Check sheet for the modelled part. Datum: model origin and axes. Units: mm. A direction names the side the tool comes from. Round coordinates to 2 decimals unless told otherwise and drop trailing zeros. Order: outer loops, then holes, each group sorted by start corner. A loop starts at its lowest first (then second) coordinate and runs counter-clockwise, first axis right, second up. Notation, with made-up numbers: (36.25, -36) -> (90.25, -36) arc R38 ccw to (90.25, 3) -> close; hole circle Ø5 at (11, 0). An arc over 180 degrees is marked (long way). Answer in a Markdown table with one row per item.
```python
from build123d import *

# Parameters (mm, degrees)
F0_W     = 130
F0_H     = 130
F1_DEPTH = 10
F3_DEPTH = 10
F4_R     = 1.5
F5_DEPTH = 10
F6_R     = 2.5
F7_DEPTH = 10
F8_R     = 3


with BuildPart() as f1:
    # F0 (on Front) → F1 (new body)
    with BuildSketch(Plane.XZ):
        Rectangle(F0_W, F0_H)
    extrude(amount=F1_DEPTH)

    # F2 (on face) → F3 (cut, through all)
    with BuildSketch(Plane.XZ.offset(10)):
        Polygon((8.8, 19.5), (-8.8, 19.5), (-19.5, 8.768557), (-19.5, -8.768557), (-8.8, -19.5), (8.8, -19.5), (19.5, -8.768557), (19.5, 8.768557), align=None)
    extrude(amount=-F3_DEPTH, mode=Mode.SUBTRACT)

    # F4 (on face) → F5 (cut, through all)
    with BuildSketch(Plane.XZ.offset(10)):
        with Locations((16, 16)):
            Circle(F4_R)
        with Locations((16, -16)):
            Circle(F4_R)
        with Locations((-16, 16)):
            Circle(F4_R)
        with Locations((-16, -16)):
            Circle(F4_R)
    extrude(amount=-F5_DEPTH, mode=Mode.SUBTRACT)

    # F6 (on face) → F7 (cut, through all)
    with BuildSketch(Plane.XZ.offset(10)):
        with Locations((52.4, 52.4)):
            Circle(F6_R)
        with Locations((52.4, -52.4)):
            Circle(F6_R)
        with Locations((-52.4, 52.4)):
            Circle(F6_R)
        with Locations((-52.4, -52.4)):
            Circle(F6_R)
    extrude(amount=-F7_DEPTH, mode=Mode.SUBTRACT)

    # F8
    f8_edges = [f1.edges().sort_by_distance(p)[0] for p in [
        (-19.5, -5, 8.768557),
        (-8.8, -5, 19.5),
        (-19.5, -5, -8.768557),
        (-8.8, -5, -19.5),
        (8.8, -5, -19.5),
        (19.5, -5, -8.768557),
        (19.5, -5, 8.768557),
        (8.8, -5, 19.5),
    ]]
    fillet(f8_edges, radius=F8_R)


solid = f1.part
```
(1) Section check D-D on y = -6.25. Give the number of separate pieces and of enclosed holes in the cut face, plus the area to 3 significant figures.
Solutions:
| item | result |
|---|---|
| separate pieces | 1 |
| enclosed holes | 9 |
| area | 15,500 mm^2 |
(2) Section check A-A on z = -52.4. Record the boundary of the cut face in (x, y), plus the area to 3 significant figures.
Solutions:
| item | result |
|---|---|
| outline | (-65, -10) -> (-54.9, -10) -> (-54.9, 0) -> (-65, 0) -> close; (-49.9, -10) -> (49.9, -10) -> (49.9, 0) -> (-49.9, 0) -> close; (54.9, -10) -> (65, -10) -> (65, 0) -> (54.9, 0) -> close |
| area | 1,200 mm^2 |
(3) Depth check by flat-ended pin: pin 1 Ø4.5 at (x, z) = (52.4, -52.4) entering from +Y. Enter the tip coordinate at first touch or a pass-through.
Solutions:
| item | result |
|---|---|
| pin 1 | through |
(4) Section check C-C on x = 52.4. Record the boundary of the cut face in (y, z), plus the area to 3 significant figures.
Solutions:
| item | result |
|---|---|
| outline | (-10, -65) -> (0, -65) -> (0, -54.9) -> (-10, -54.9) -> close; (-10, -49.9) -> (0, -49.9) -> (0, 49.9) -> (-10, 49.9) -> close; (-10, 54.9) -> (0, 54.9) -> (0, 65) -> (-10, 65) -> close |
| area | 1,200 mm^2 |
(5) Section check B-B on z = -4. Record the boundary of the cut face in (x, y).
Solutions:
| item | result |
|---|---|
| outline | (-65, -10) -> (-19.5, -10) -> (-19.5, 0) -> (-65, 0) -> close; (19.5, -10) -> (65, -10) -> (65, 0) -> (19.5, 0) -> close |
(6) Tool access check on faces 1 (the flat face through (65, -5, -1)), 2 (the flat face through (-19.5, -5, 0)). Record the directions out of +Z, -Z, +X, -X, +Y, -Y that give a thin tool (end or side, any length) a straight path to the whole face; none if there is none.
Solutions:
| item | result |
|---|---|
| face 1 | +Z, -Z, +X, +Y, -Y |
| face 2 | +Y, -Y |
(7) Draft check along Z on faces 3 (the flat face through (-15, -10, -14)), 4 (the cylindrical face through (54.71, -5.07, 51.44)), 5 (the flat face through (0, -5, -19.5)), 6 (the flat face through (-1, -5, -65)). Enter one of: pulls with the +Z half, pulls with the -Z half, needs draft (parallel to the pull), parting line crosses it, or undercut.
Solutions:
| item | result |
|---|---|
| face 3 | needs draft |
| face 4 | undercut |
| face 5 | undercut |
| face 6 | pulls with the -Z half |
(8) Scan lines: probe 1 along Z at (x, y) = (52.4, -6); probe 2 along Z at (x, y) = (6, -5.25); probe 3 along Z at (x, y) = (-16, -5.25). Record each from-to range of solid material in increasing order. Write a range as from..to.
Solutions:
| item | result |
|---|---|
| probe 1 | -65..-54.9, -49.9..49.9, 54.9..65 |
| probe 2 | -65..-19.5, 19.5..65 |
| probe 3 | -65..-17.5, -14.5..-12.28, 12.28..14.5, 17.5..65 |
